For this review, take the finished solid that the model builds, in its own axes (mm). Coordinates: 2 decimals unless noted, no trailing zeros. Write each loop counter-clockwise with the first axis right and the second up, starting at its lowest first coordinate (ties: lowest second). Pieces come first, ordered by that corner, then holes.
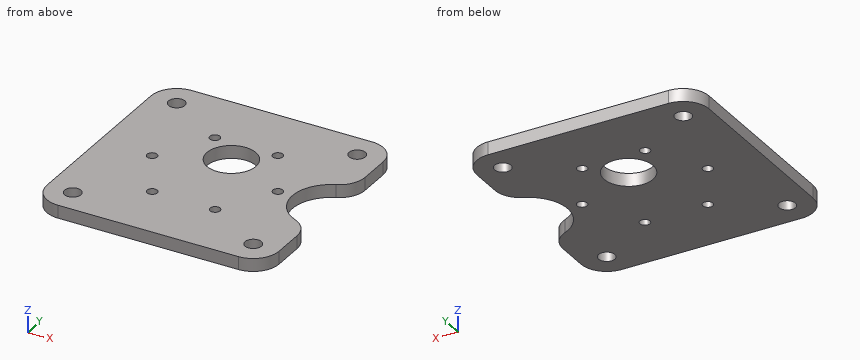
```python
from build123d import *

# Parameters (mm, degrees)
SKETCH1_R           = 2.0193
SKETCH1_R_2         = 1.2446
SKETCH1_R_3         = 6.0325
BOSS_EXTRUDE1_DEPTH = 1.5875
FILLET2_R           = 6.35


with BuildPart() as part:
    # Sketch1 → Boss-Extrude1 (new, symmetric)
    with BuildSketch(Plane.XY):
        with BuildLine():
            Line((28.575, 28.575), (-28.575, 28.575))
            Line((-28.575, 28.575), (-28.575, -28.575))
            Line((-28.575, -28.575), (28.575, -28.575))
            Line((28.575, -28.575), (28.575, -9.525))
            ThreePointArc((28.575, -9.525), (19.05, 0), (28.575, 9.525))
            Line((28.575, 9.525), (28.575, 28.575))
        make_face()
        with Locations((-22.225, -22.225)):
            Circle(SKETCH1_R, mode=Mode.SUBTRACT)
        with Locations((-7.747, -13.418197606)):
            Circle(SKETCH1_R_2, mode=Mode.SUBTRACT)
        with Locations((22.225, -22.225)):
            Circle(SKETCH1_R, mode=Mode.SUBTRACT)
        with Locations((7.747, -13.418197606)):
            Circle(SKETCH1_R_2, mode=Mode.SUBTRACT)
        with Locations((15.494, 0)):
            Circle(SKETCH1_R_2, mode=Mode.SUBTRACT)
        with Locations((-15.494, 0)):
            Circle(SKETCH1_R_2, mode=Mode.SUBTRACT)
        with Locations((-7.747, 13.418197606)):
            Circle(SKETCH1_R_2, mode=Mode.SUBTRACT)
        with Locations((-22.225, 22.225)):
            Circle(SKETCH1_R, mode=Mode.SUBTRACT)
        with Locations((0, 7.0104)):
            Circle(SKETCH1_R_3, mode=Mode.SUBTRACT)
        with Locations((7.747, 13.418197606)):
            Circle(SKETCH1_R_2, mode=Mode.SUBTRACT)
        with Locations((22.225, 22.225)):
            Circle(SKETCH1_R, mode=Mode.SUBTRACT)
    extrude(amount=BOSS_EXTRUDE1_DEPTH, both=True)

    # Fillet2
    fillet2_edges = [part.edges().sort_by_distance(p)[0] for p in [
        (28.575, -9.525, 0),
        (28.575, -28.575, 0),
        (-28.575, -28.575, 0),
        (-28.575, 28.575, 0),
        (28.575, 28.575, 0),
        (28.575, 9.525, 0),
    ]]
    fillet(fillet2_edges, radius=FILLET2_R)


solid = part.part
```
1) Consider section A-A (y = 0). Count the separate pieces of the cut face and the enclosed holes in it, then the cut area to 3 significant figures.
2) Consider section D-D (y = 21). Give the boundary of the cut face in (x, z) (1 decimal).
3) For L1, parallel to X at y = -13.5, z = 0.05 (3 decimals); L2, parallel to Y at x = -20.5, z = 1.1 (3 decimals); L3, parallel to Y at x = 22, z = 1.05 (3 decimals), list the stretches that pass through material, from the lowest coordinate up.
4) Clearance check with a flat-ended pin moving along its axis: P1, Ø1.5, axis at x = 7.75, y = -13.42, coming from the +Z side. State where the tip first meets the part, or that it passes through.
5) Consider section B-B (x = 0). Give the boundary of the cut face in (y, z) (1 decimal).
Results:
1. separate pieces: 3
1. enclosed holes: 0
1. area: 135 mm2
2. outline: (-28.6, -1.6) - (-23.8, -1.6) - (-23.8, 1.6) - (-28.6, 1.6) - close; (-20.6, -1.6) - (20.6, -1.6) - (20.6, 1.6) - (-20.6, 1.6) - close; (23.8, -1.6) - (28.6, -1.6) - (28.6, 1.6) - (23.8, 1.6) - close
3. L1: x = -28.575 to -8.989, -6.505 to 6.505, 8.989 to 28.488
3. L2: y = -28.575 to -23.275, -21.175 to 21.175, 23.275 to 28.575
3. L3: y = -28.575 to -24.232, -20.218 to -6.892, 6.892 to 20.218, 24.232 to 28.575
4. P1: passes through
5. outline: (-28.6, -1.6) - (1, -1.6) - (1, 1.6) - (-28.6, 1.6) - close; (13, -1.6) - (28.6, -1.6) - (28.6, 1.6) - (13, 1.6) - close
